Geometry check sheet. Reference: the model listing, model coordinates, mm. Face numbers are marked on the shaded views. A direction names the side the tool comes from. Round coordinates to 2 decimals unless told otherwise and drop trailing zeros. Loops run counter-clockwise (first coordinate to the right, second up) from the corner with the lowest first, then second, coordinate; pieces in that order, holes last. Notation, with made-up numbers: (58.25, 2.25) -> (84.25, 2.25) arc R26 ccw to (84.25, 41.25) -> close; hole circle Ø7 at (42.5, 6.5). An arc over 180 degrees is marked (long way). Use a Markdown table: item, result. Add a question column.
Q1. Release check for a two-part mould opening along Z. For the marked faces 3, 4 and 5 record: released by +Z, released by -Z, zero draft, split by the parting line, or undercut.
Q2. Sectioned sample at B-B, the plane y = -19.5. Enter the section's corners in (x, z).
Q3. Sectioned sample at A-A, the plane x = -35. Enter the section's corners in (y, z), then the cut area to 3 significant figures.
Q4. Sectioned sample at C-C, the plane z = 6.25. Enter the section's corners in (x, y).
Q5. Sectioned sample at D-D, the plane x = -14.4. Enter the section's corners in (y, z), then the cut area to 3 significant figures.
Q6. Material ranges on L1, parallel to Y at x = -26, z = 21.75; L2, parallel to Z at x = 43.5, y = -6.5; L3, parallel to X at y = -16, z = 13.75, recorded low to high.
Q7. Set-up check for the marked faces 1 and 2: record each of +Z, -Z, +X, -X, +Y, -Y from which the full face is reachable in a straight line by a thin tool's end or side.
Q8. Gauge pin test, flat ends, axial feed: P1, Ø2.5, axis at x = -5.5, y = 24, coming from the +Z side; P2, Ø1.8, axis at x = 44.5, y = 8, coming from the -Z side; P3, Ø1, axis at x = 28.5, y = -2.5, coming from the +Z side; P4, Ø1, axis at x = -8.5, y = -24, coming from the +Z side. Record the tip position at first contact, or that the pin passes through.
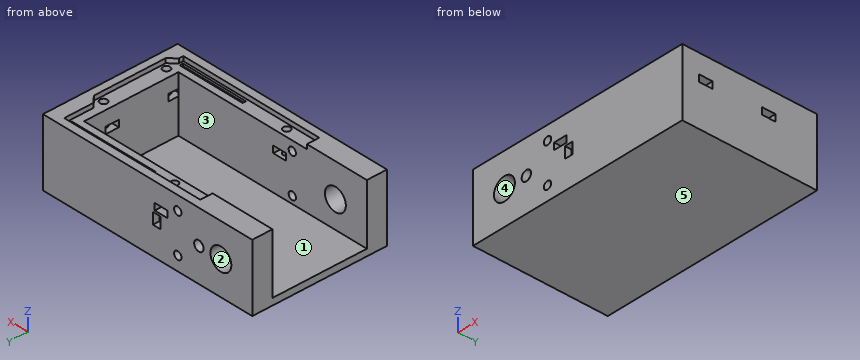
```python
from build123d import *

# Parameters (mm, degrees)
F1_DEPTH  = 30
F0_W      = 90
F0_H      = 42
F2_DEPTH  = 3
F3_R      = 5
F3_R_2    = 1.75
F4_DEPTH  = 9
F3_R_3    = 2.25
F3_W      = 3.5
F3_H      = 5
F5_DEPTH  = 3
F7_W      = 40
F7_H      = 1.5
F7_W_2    = 30
F8_DEPTH  = 3
F7_R      = 1.6
F9_DEPTH  = 2
F10_DEPTH = 15
F11_W     = 6
F11_H     = 3
F12_DEPTH = 9
F13_W     = 6
F13_H     = 3
F14_DEPTH = 9
F15_W     = 6
F15_H     = 3
F16_DEPTH = 10


with BuildPart() as f1:
    # F0 (on Top) → F1 (new body)
    with BuildSketch(Plane.XY):
        Polygon((50, 30), (-50, 30), (-50, 21), (40, 21), (40, -21), (-50, -21), (-50, -30), (50, -30), align=None)
    extrude(amount=F1_DEPTH)

    # F0 (on Top) → F2 (join)
    with BuildSketch(Plane.XY):
        with Locations((-5, 0)):
            Rectangle(F0_W, F0_H)
    extrude(amount=F2_DEPTH)

    # F3 (on face) → F4 (cut, through all)
    with BuildSketch(Plane.XZ.offset(30)):
        with Locations((-35, 15)):
            Circle(F3_R)
        with Locations((-14.4, 23.75)):
            Circle(F3_R_2)
        with Locations((-14.4, 6.25)):
            Circle(F3_R_2)
    extrude(amount=-F4_DEPTH, mode=Mode.SUBTRACT)

    # F3 (on face) → F5 (cut)
    with BuildSketch(Plane.XZ.offset(30)):
        with Locations((-24.5, 15)):
            Circle(F3_R_3)
        with Locations((-4.3, 15)):
            Rectangle(F3_W, F3_H)
    extrude(amount=-F5_DEPTH, mode=Mode.SUBTRACT)

    # F6: F1 across plane


with BuildPart() as f1_1:
    add(f1.part)
    add(f1.part.mirror(Plane.XZ), mode=Mode.INTERSECT)

    # F7 (on face) → F8 (cut)
    with BuildSketch(Plane.XY.offset(30)):
        with Locations((22.6103741318, 24.75)):
            Rectangle(F7_W, F7_H)
        with Locations((27.6103741318, -24.75)):
            Rectangle(F7_W_2, F7_H)
    extrude(amount=-F8_DEPTH, mode=Mode.SUBTRACT)

    # F7 (on face) → F9 (cut)
    with BuildSketch(Plane.XY.offset(30)):
        Polygon((43.6103741318, 26.5), (-21.3896258682, 26.5), (-21.3896258682, -26.5), (43.6103741318, -26.5), (43.6103741318, -24.5), (46.6103741318, -21.5), (46.6103741318, 10.5), (43.6103741318, 13.5), align=None)
        with Locations((-8.2896258682, -24.2)):
            Circle(F7_R, mode=Mode.SUBTRACT)
        with Locations((27.6103741318, -24.75)):
            Rectangle(F7_W_2, F7_H, mode=Mode.SUBTRACT)
        with Locations((44.1103741318, -19.5)):
            Circle(F7_R, mode=Mode.SUBTRACT)
        with Locations((-6.3896258682, 24)):
            Circle(F7_R, mode=Mode.SUBTRACT)
        with Locations((44.1103741318, 8.5)):
            Circle(F7_R, mode=Mode.SUBTRACT)
        with Locations((22.6103741318, 24.75)):
            Rectangle(F7_W, F7_H, mode=Mode.SUBTRACT)
    extrude(amount=-F9_DEPTH, mode=Mode.SUBTRACT)

    # F10 (cut): faces of the model
    f10_faces = [f1_1.faces().sort_by_distance(p)[0] for p in [
        (-6.3896258682, 24, 30),
        (44.1103741318, 8.5, 30),
        (44.1103741318, -19.5, 30),
        (-8.2896258682, -24.2, 30),
    ]]
    extrude(f10_faces, amount=-F10_DEPTH, mode=Mode.SUBTRACT)

    # F11 (on face) → F12 (cut, through all)
    with BuildSketch(Plane.XZ.offset(-21)):
        with Locations((-6.3896258682, 20)):
            Rectangle(F11_W, F11_H)
    extrude(amount=-F12_DEPTH, mode=Mode.SUBTRACT)

    # F13 (on face) → F14 (cut, through all)
    with BuildSketch(Plane(origin=(0, -21, 0), x_dir=(-1, 0, 0), z_dir=(0, 1, 0))):
        with Locations((8.2896258682, 20)):
            Rectangle(F13_W, F13_H)
    extrude(amount=-F14_DEPTH, mode=Mode.SUBTRACT)

    # F15 (on face) → F16 (cut, through all)
    with BuildSketch(Plane(origin=(40, 0, 0), x_dir=(0, -1, 0), z_dir=(-1, 0, 0))):
        with Locations((-8.5, 20)):
            Rectangle(F15_W, F15_H)
        with Locations((19.5, 20)):
            Rectangle(F15_W, F15_H)
    extrude(amount=-F16_DEPTH, mode=Mode.SUBTRACT)


solid = f1_1.part
```
Values:
| question | item | result |
|---|---|---|
| 1 | face 3 | zero draft |
| 1 | face 4 | undercut |
| 1 | face 5 | released by -Z |
| 2 | outline | (-50, 0) -> (50, 0) -> (50, 18.5) -> (45.71, 18.5) -> (45.71, 15) -> (42.51, 15) -> (42.51, 18.5) -> (40, 18.5) -> (40, 3) -> (-50, 3) -> close; (40, 21.5) -> (42.51, 21.5) -> (42.51, 28) -> (40, 28) -> close; (45.71, 21.5) -> (50, 21.5) -> (50, 30) -> (46.61, 30) -> (46.61, 28) -> (45.71, 28) -> close |
| 3 | outline | (-30, 0) -> (30, 0) -> (30, 10) -> (21, 10) -> (21, 3) -> (-21, 3) -> (-21, 10) -> (-30, 10) -> close; (-30, 20) -> (-21, 20) -> (-21, 30) -> (-30, 30) -> close; (21, 20) -> (30, 20) -> (30, 30) -> (21, 30) -> close |
| 3 | area | 486 mm^2 |
| 4 | outline | (-50, -30) -> (-16.15, -30) -> (-16.15, -21) -> (-50, -21) -> close; (-50, 21) -> (-16.15, 21) -> (-16.15, 30) -> (-50, 30) -> close; (-12.65, -30) -> (50, -30) -> (50, 30) -> (-12.65, 30) -> (-12.65, 21) -> (40, 21) -> (40, -21) -> (-12.65, -21) -> close |
| 5 | outline | (-30, 0) -> (30, 0) -> (30, 4.5) -> (21, 4.5) -> (21, 3) -> (-21, 3) -> (-21, 4.5) -> (-30, 4.5) -> close; (-30, 8) -> (-21, 8) -> (-21, 22) -> (-30, 22) -> close; (-30, 25.5) -> (-21, 25.5) -> (-21, 28) -> (-26.5, 28) -> (-26.5, 30) -> (-30, 30) -> close; (21, 8) -> (30, 8) -> (30, 22) -> (21, 22) -> close; (21, 25.5) -> (30, 25.5) -> (30, 30) -> (26.5, 30) -> (26.5, 28) -> (21, 28) -> close |
| 5 | area | 518 mm^2 |
| 6 | L1 | -30 to -21, 21 to 30 |
| 6 | L2 | 0 to 28 |
| 6 | L3 | 40 to 50 |
| 7 | face 1 | +Z, -X |
| 7 | face 2 | +Y, -Y |
| 8 | P1 | z = 28 |
| 8 | P2 | z = 0 |
| 8 | P3 | z = 3 |
| 8 | P4 | z = 15 |
